Check sheet for the drawn part. Datum: minimum x, y, z corner. Units: mm. Round coordinates to 2 decimals unless told otherwise and drop trailing zeros. Order: outer loops, then holes, each group sorted by start corner. A loop starts at its lowest first (then second) coordinate and runs counter-clockwise, first axis right, second up. Notation, with made-up numbers: (-37, 47.25) - (8, 47.25) arc R34 cw to (8, 82.25) - close; hole circle Ø4 at (46, 9). An arc over 180 degrees is marked (long way). Write each question's results on one line, items separated by ' | '.
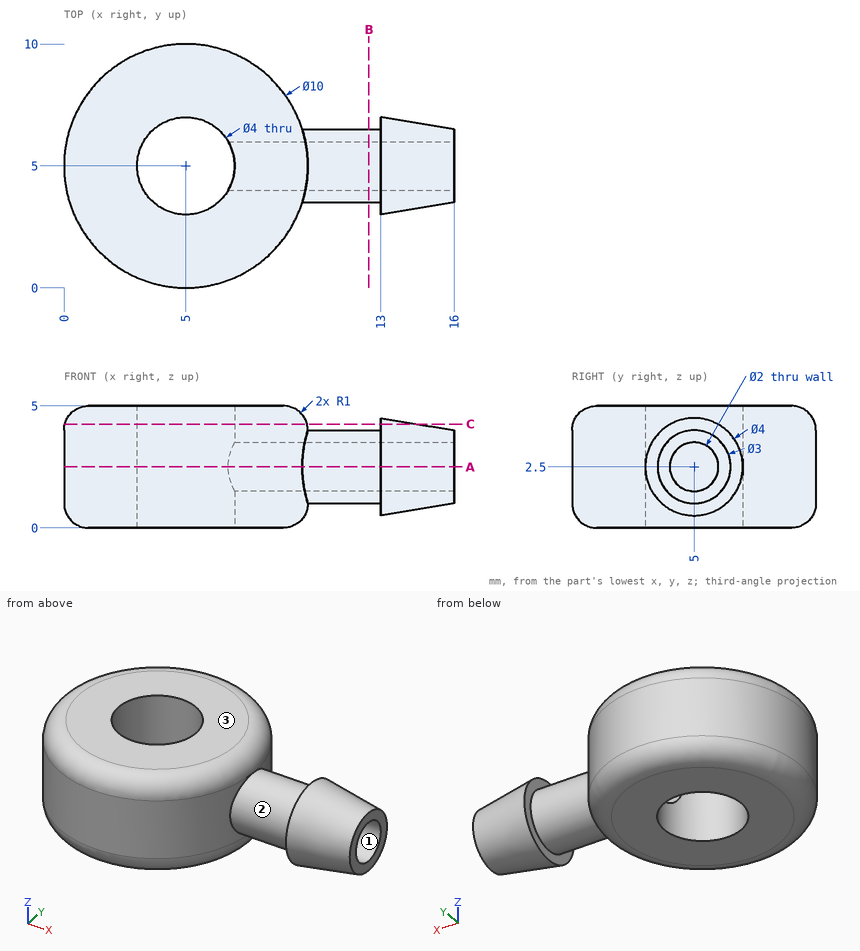
(1) Depth check by flat-ended pin: pin 1 Ø3.5 at (x, y) = (5, 5) entering from +Z; pin 2 Ø1.2 at (y, z) = (5, 2.5) entering from +X; pin 3 Ø1.5 at (y, z) = (9, 1.5) entering from -X. Enter the tip coordinate at first touch or a pass-through.
Answers follow:
pin 1: through | pin 2: x = 3.09 | pin 3: x = 1.2
(2) Draft check along Y on the marked faces 1, 2 and 3. Enter one of: released by +Y, released by -Y, zero draft, split by the parting line, or undercut.
Answers follow:
face 1: undercut | face 2: split by the parting line | face 3: zero draft
(3) Section check A-A (z = 2.5). Record the cut outline in (x, y), then the cut area to 3 significant figures.
Answers follow:
outline: (6.73, 4) arc R2 cw (long way) to (6.73, 6) - (16, 6) - (16, 6.5) - (13, 7) - (13, 6.5) - (9.77, 6.5) arc R5 ccw (long way) to (9.77, 3.5) - (13, 3.5) - (13, 3) - (16, 3.5) - (16, 4) - close | area: 67.5 mm²
(4) Section check C-C (z = 4.25). Give the number of separate pieces and of enclosed holes in the cut face, then the cut area to 3 significant figures.
Answers follow:
separate pieces: 2 | enclosed holes: 1 | area: 66.9 mm²
(5) Material ranges on line 1 (Y direction, x = 5, z = 3.3); line 2 (Y direction, x = 4.5, z = 0.25); line 3 (X direction, y = 4.5, z = 0.5), recorded low to high.
Answers follow:
line 1: 0 to 3, 7 to 10 | line 2: 0.37 to 3.06, 6.94 to 9.63 | line 3: 0.16 to 3.06, 6.94 to 9.84
(6) Section check B-B (x = 12.5). Record the cut outline in (y, z), then the cut area to 3 significant figures.
Answers follow:
outline: circle Ø3 at (5, 2.5); hole circle Ø2 at (5, 2.5) | area: 3.93 mm²
